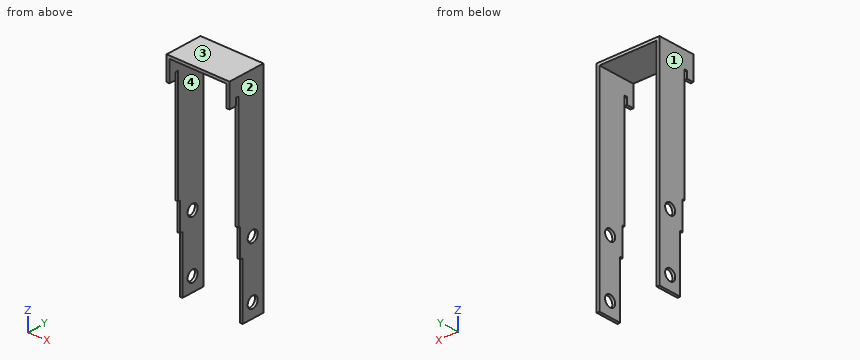
```python
from build123d import *

# Parameters (mm, degrees)
SKETCH1_R           = 4
BOSS_EXTRUDE1_DEPTH = 2
SKETCH2_W           = 45
SKETCH2_H           = 27
BOSS_EXTRUDE2_DEPTH = 2


with BuildPart() as part:
    # Sketch1 → Boss-Extrude1 (new body)
    with BuildSketch(Plane.YZ):
        Polygon((8.5, -10), (8.5, 140), (-18.5, 140), (-18.5, 125), (-13.5, 125), (-13.5, 130), (-11.5, 130), (-11.5, 50.152793502), (-10, 50.152793502), (-10, 30.152793502), (-8, 30.152793502), (-8, -10), align=None)
        Circle(SKETCH1_R, mode=Mode.SUBTRACT)
        with Locations((0, 40.152793502)):
            Circle(SKETCH1_R, mode=Mode.SUBTRACT)
    extrude(amount=-BOSS_EXTRUDE1_DEPTH)


with BuildPart() as body_2:
    # Mirror2: mirrored copy
    add(part.part.mirror(Plane.ZY.offset(22.5)))


with BuildPart() as part_1:
    add(part.part)

    add(body_2.part)  # Boss-Extrude2 merges body 2
    # Sketch2 → Boss-Extrude2 (add)
    with BuildSketch(Plane.XY.offset(140)):
        with Locations((-22.5, -5)):
            Rectangle(SKETCH2_W, SKETCH2_H)
    extrude(amount=BOSS_EXTRUDE2_DEPTH)


solid = part_1.part
```
Input: part model. Units: mm. Frame: model coordinates. Face numbers are marked on the shaded views. Round coordinates to 2 decimals unless told otherwise and drop trailing zeros. Loops run counter-clockwise (first coordinate to the right, second up) from the corner with the lowest first, then second, coordinate; pieces in that order, holes last. Notation, with made-up numbers: (85.25, 74) - (129.25, 74) arc R18 ccw to (129.25, 86) - close; hole circle Ø5 at (2, 66.25). An arc over 180 degrees is marked (long way). One line per item, written item: value. Start each with the question number.
(1) Section C-C, the plane z = 0. Return loops of the section in (x, y), plus the area to 3 significant figures.
(2) Section A-A, the plane y = 0. Return loops of the section in (x, z).
(3) Ray query, line 1 (Z direction, x = -1.4, y = 0); line 2 (X direction, y = 6.25, z = 14); line 3 (Z direction, x = -17, y = -9.5). Return the intervals inside material, ascending. Write a range as [from, to].
(4) Draft query along X for the marked faces 1, 2, 3 and 4. Return one class per face: +X half, -X half, draft (parallel to the pull), parting line (faces both ways), or undercut.
(5) Contact query for flat-ended pins moving along their axis: P1, Ø1, axis at x = -43.5, y = -15, coming from the -Z side; P2, Ø4, axis at x = -11, y = -11.5, coming from the -Z side; P3, Ø0.6, axis at x = -44, y = -12, coming from the -Z side; P4, Ø5, axis at y = 0, z = 0, coming from the +X side. Output: stop coordinate, or through.
(6) Section D-D, the plane y = -16. Return loops of the section in (x, z).
(7) Section B-B, the plane z = 58.5. Return loops of the section in (x, y).
Results below:
1. outline: (-45, -8) - (-43, -8) - (-43, -4) - (-45, -4) - close; (-45, 4) - (-43, 4) - (-43, 8.5) - (-45, 8.5) - close; (-2, -8) - (0, -8) - (0, -4) - (-2, -4) - close; (-2, 4) - (0, 4) - (0, 8.5) - (-2, 8.5) - close
1. area: 34.0 mm^2
2. outline: (-45, -10) - (-43, -10) - (-43, -4) - (-45, -4) - close; (-45, 4) - (-43, 4) - (-43, 36.15) - (-45, 36.15) - close; (-45, 44.15) - (-43, 44.15) - (-43, 140) - (-2, 140) - (-2, 44.15) - (0, 44.15) - (0, 142) - (-45, 142) - close; (-2, -10) - (0, -10) - (0, -4) - (-2, -4) - close; (-2, 4) - (0, 4) - (0, 36.15) - (-2, 36.15) - close
3. line 1: [-10, -4], [4, 36.15], [44.15, 142]
3. line 2: [-45, -43], [-2, 0]
3. line 3: [140, 142]
4. face 1: -X half
4. face 2: +X half
4. face 3: draft
4. face 4: undercut
5. P1: z = 125
5. P2: z = 140
5. P3: z = 130
5. P4: through
6. outline: (-45, 125) - (-43, 125) - (-43, 140) - (-2, 140) - (-2, 125) - (0, 125) - (0, 142) - (-45, 142) - close
7. outline: (-45, -11.5) - (-43, -11.5) - (-43, 8.5) - (-45, 8.5) - close; (-2, -11.5) - (0, -11.5) - (0, 8.5) - (-2, 8.5) - close
